Autodesk Inventor part; units mm, degrees
ref_plane "YZ Plane" through (0, 0, 0) normal (1, 0, 0) x (0, 1, 0)
ref_plane "XZ Plane" through (0, 0, 0) normal (0, 1, 0) x (-1, 0, 0)
ref_plane "XY Plane" through (0, 0, 0) normal (0, 0, 1) x (1, 0, 0)
sketch "Skizze1" plane through (0, 0, 0) normal (1, 0, 0) x (0, 1, 0)
  line L0 (-4.25, -6.5) -> (4.25, -6.5)
  line L1 (4.25, -6.5) -> (4.25, 6.5)
  line L2 (4.25, 6.5) -> (-4.25, 6.5)
  line L3 (-4.25, 6.5) -> (-4.25, -6.5)
  line L4 (-4.25, -6.5) -> (4.25, 6.5) construction
  line L5 (4.25, -6.5) -> (-4.25, 6.5) construction
  point P0 (0, 0)
  dimension "d0" = 8.5
  dimension "d1" = 13
extrude "Extrusion1" add sketch "Skizze1" along normal blind 2.5
sketch "Skizze3" plane through (0, 0, 0) normal (0, 1, 0) x (-1, 0, 0)
  line L0 (-1.0667, -6.5) -> (-0.0476, -3.7)
  line L1 (-0.0476, -3.7) -> (3.1717, -7.0921)
  line L2 (3.1717, -7.0921) -> (1.0847, -12.4156)
  line L3 (1.0847, -12.4156) -> (-1.0667, -6.5)
  line L4 (0, -6.5) -> (-2.5, -6.5)
  line L5 (0, -6.5) -> (0, 6.5)
  point P0 (0, 0)
  dimension "d11" = 2.8
  dimension "d12" = 20
extrude "Extrusion3" cut sketch "Skizze3" along normal mid plane 10.75
fillet "Rundung1" radius 2 4 edges at (1.25, 4.25, 6.5) (1.25, -4.25, 6.5) (1.7834, 4.25, -6.5) (1.7834, -4.25, -6.5)
sketch "Skizze2" plane through (0, 0, 0) normal (-1, 0, 0) x (0, 0, 1)
  circle A0 centre (2.5, 0) radius 2.4
  line L0 (6.5, 2.25) -> (6.5, -2.25)
  point P0 (0, 0)
  dimension "d6" = 4.8
  dimension "d13" = 4
extrude "Extrusion2" cut sketch "Skizze2" against normal blind 10.75
properties part number "P_PIN"
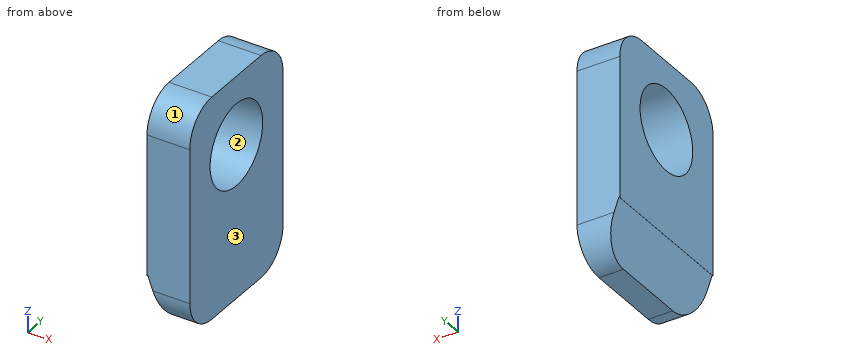
Geometry check sheet. Reference: the model listing, model coordinates, mm. Face numbers are marked on the shaded views. Give positions to 0.01 mm unless a question says otherwise; leave off trailing zeros. Loops run counter-clockwise (first coordinate to the right, second up) from the corner with the lowest first, then second, coordinate; pieces in that order, holes last. Notation, with made-up numbers: M 21.25,68.5 L 65.25,68.5 A12 ccw 65.25,86.5 Z; hole C 21.5,47 d8. An arc over 180 degrees is marked long. Answer as a JSON object with one key per item and string values. Group by question number.
Item 1: Material ranges on L1, parallel to Y at x = 0.75, z = 2.5; L2, parallel to Y at x = 0.5, z = 0.5; L3, parallel to Z at x = 1.2, y = -1.25, recorded low to high.
Item 2: Sectioned sample at A-A on x = 1.8. Record the boundary of the cut face in (y, z), plus the area to 3 significant figures.
Item 3: Mould release check, pull along Z, two halves, no side actions. Record for the marked faces 1, 2 and 3: pulls with the +Z half, pulls with the -Z half, needs draft (parallel to the pull), parting line crosses it, or undercut.
Item 4: Sectioned sample at C-C on z = 2.5. Record the boundary of the cut face in (x, y).
Item 5: Sectioned sample at B-B on y = -0.75. Record the boundary of the cut face in (x, z), plus the area to 3 significant figures.
Item 6: Sectioned sample at D-D on y = 1. Record the boundary of the cut face in (x, z).
Findings below:
{
 "1": {"L1": "-4.25 to -2.4, 2.4 to 4.25", "L2": "-4.25 to -1.33, 1.33 to 4.25", "L3": "-6.5 to 0.45, 4.55 to 6.5"},
 "2": {"outline": "M -4.25,-4.5 A2 ccw -2.25,-6.5 L 2.25,-6.5 A2 ccw 4.25,-4.5 L 4.25,4.5 A2 ccw 2.25,6.5 L -2.25,6.5 A2 ccw -4.25,4.5 Z; hole C 0,2.5 d4.8", "area": "89.0 mm2"},
 "3": {"face 1": "pulls with the +Z half", "face 2": "undercut", "face 3": "needs draft"},
 "4": {"outline": "M 0,-4.25 L 2.5,-4.25 L 2.5,-2.4 L 0,-2.4 Z; M 0,2.4 L 2.5,2.4 L 2.5,4.25 L 0,4.25 Z"},
 "5": {"outline": "M 0,-3.75 L 0.05,-3.7 L 1.07,-6.5 L 2.5,-6.5 L 2.5,0.22 L 0,0.22 Z; M 0,4.78 L 2.5,4.78 L 2.5,6.5 L 0,6.5 Z", "area": "19.5 mm2"},
 "6": {"outline": "M 0,-3.75 L 0.05,-3.7 L 1.07,-6.5 L 2.5,-6.5 L 2.5,0.32 L 0,0.32 Z; M 0,4.68 L 2.5,4.68 L 2.5,6.5 L 0,6.5 Z"}
}
